```python
from build123d import *

# Parameters (mm, degrees)
F0_W         = 13
F0_H         = 24
F1_DEPTH     = 5
F0_W_2       = 18
F0_H_2       = 5
F2_W         = 83
F2_H         = 80
F3_DEPTH     = 2
F4_W         = 9
F4_H         = 17
F5_DEPTH     = 5
F6_W         = 12
F6_H         = 6
F7_DEPTH     = 10
F8_W         = 12
F8_H         = 4
F9_DEPTH     = 10
F10_T1_DEPTH = 9


# Not quite as in the source:
# - a fillet or chamfer that OpenCascade refuses, or shapes differently, is made with other operations: its cross-section is extruded or revolved along the edge and cut away or added


with BuildPart() as f1:
    # F0 (on Top) → F1 (new body)
    with BuildSketch(Plane.XY):
        Polygon((-19.7103468106, 42.4778270721), (-46.7103468106, 42.4778270721), (-46.7103468106, -37.5221729279), (36.2896531894, -37.5221729279), (36.2896531894, 42.4778270721), (22.2896531894, 42.4778270721), (22.2896531894, 37.4778270721), (31.2896531894, 37.4778270721), (31.2896531894, -32.5221729279), (-23.7103468106, -32.5221729279), (-23.7103468106, 37.4778270721), (-19.7103468106, 37.4778270721), align=None)
        with Locations((-35.2103468106, -3.5221729279)):
            Rectangle(F0_W, F0_H, mode=Mode.SUBTRACT)
    extrude(amount=F1_DEPTH)



with BuildPart() as f1b:
    # F0 (on Top) → F1, piece 2 (new body)
    with BuildSketch(Plane.XY):
        with Locations((-0.7103468106, 39.9778270721)):
            Rectangle(F0_W_2, F0_H_2)
    extrude(amount=F1_DEPTH)


with BuildPart() as f1_1:
    add(f1.part)

    add(f1b.part)  # F3 merges F1b
    # F2 (on face) → F3 (join)
    with BuildSketch(Plane(origin=(0, 0, 0), x_dir=(1, 0, 0), z_dir=(0, 0, -1))):
        with Locations((-5.2103468106, -2.4778270721)):
            Rectangle(F2_W, F2_H)
    extrude(amount=F3_DEPTH)

    # F4 (on face) → F5 (cut)
    with BuildSketch(Plane.XY.offset(5)):
        with Locations((-35.2103468106, -24.0221729279)):
            Rectangle(F4_W, F4_H)
    extrude(amount=-F5_DEPTH, mode=Mode.SUBTRACT)

    # F6 (on face) → F7 (join)
    with BuildSketch(Plane.XY.offset(5)):
        with Locations((-35.2103468106, 11.4778270721)):
            Rectangle(F6_W, F6_H)
    extrude(amount=F7_DEPTH)

    # F8 (on face) → F9 (join)
    with BuildSketch(Plane.XY.offset(5)):
        with Locations((-35.2103468106, -18.5221729279)):
            Rectangle(F8_W, F8_H)
    extrude(amount=F9_DEPTH)

    # F10: fillet of radius 12 on 1 edges, made by hand

    # F10_s2 → F10_t1 (join)
    with BuildSketch(Plane.YZ.offset(-39.7103468106)):
        with BuildLine():
            ThreePointArc((-32.5221729279, 5), (-28.2526041581, 1.322921748), (-22.775378583, 0))
            Line((-22.775378583, 0), (-32.5221729279, 0))
            Line((-32.5221729279, 0), (-32.5221729279, 5))
        make_face()
    extrude(amount=F10_T1_DEPTH)


solid = f1_1.part
```
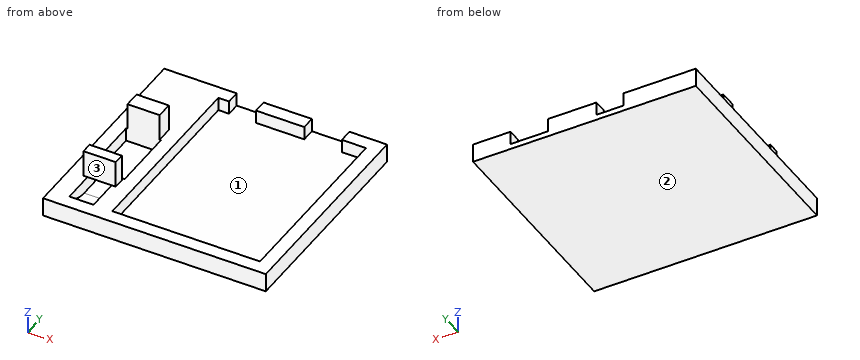
Here's how the part is built. I have some questions about the finished solid (model axes, mm). Face numbers are marked on the shaded views. Coordinates: 2 decimals unless noted, no trailing zeros. Order: outer loops, then holes, each group sorted by start corner. A loop starts at its lowest first (then second) coordinate and runs counter-clockwise, first axis right, second up. Notation, with made-up numbers: (84, 68) - (117, 68) arc R10 ccw to (117, 76) - close; hole circle Ø10 at (46, -32). An arc over 180 degrees is marked (long way). One line per question, with ' | ' between items.
(1) If we mould it in two halves opening along Y, with no side actions, what happens to the marked faces 1, 2 and 3? For each: pulls with the +Y half, pulls with the -Y half, needs draft (parallel to the pull), parting line crosses it, or undercut.
Report:
face 1: undercut | face 2: needs draft | face 3: pulls with the -Y half
(2) Suppose I cut it at C-C on y = 16. List the corners of the cut face in (x, z) for me.
Report:
outline: (-46.71, -2) - (36.29, -2) - (36.29, 5) - (31.29, 5) - (31.29, 0) - (-23.71, 0) - (-23.71, 5) - (-46.71, 5) - close
(3) Suppose I cut it at A-A on y = -17.5. List the corners of the cut face in (x, z) for me.
Report:
outline: (-46.71, -2) - (36.29, -2) - (36.29, 5) - (31.29, 5) - (31.29, 0) - (-23.71, 0) - (-23.71, 5) - (-29.21, 5) - (-29.21, 15) - (-41.21, 15) - (-41.21, 5) - (-46.71, 5) - close; hole (-39.71, 0) - (-30.71, 0) - (-30.71, 5) - (-39.71, 5) - close
(4) Suppose I cut it at D-D on x = 0. List the corners of the cut face in (y, z) for me.
Report:
outline: (-37.52, -2) - (42.48, -2) - (42.48, 5) - (37.48, 5) - (37.48, 0) - (-32.52, 0) - (-32.52, 5) - (-37.52, 5) - close
(5) Suppose I cut it at B-B on z = 6. List the corners of the cut face in (x, y) for me.
Report:
outline: (-41.21, -20.52) - (-29.21, -20.52) - (-29.21, -16.52) - (-41.21, -16.52) - close; (-41.21, 8.48) - (-29.21, 8.48) - (-29.21, 14.48) - (-41.21, 14.48) - close
(6) Will these pins go through, and if not, where does the flat tip stop? pin 1 (1.2 mm diameter, centred on y = -18, z = 8.5, fed in from +X); pin 2 (8 mm diameter, centred on x = -33.5, z = 10.5, fed in from +Y); pin 3 (2 mm diameter, centred on x = -11.5, y = 12, fed in from +Z).
Report:
pin 1: stops at x = -29.21 | pin 2: stops at y = 14.48 | pin 3: stops at z = 0
(7) If I drill on L1, parallel to X at y = -6, z = 1.25; L2, parallel to X at y = -19, z = 4; L3, parallel to X at y = 9, z = 1.75, over which ranges is the centre line in solid material (lowest first)?
Report:
L1: x = -46.71 to -41.71, -28.71 to -23.71, 31.29 to 36.29 | L2: x = -46.71 to -39.71, -30.71 to -23.71, 31.29 to 36.29 | L3: x = -46.71 to -23.71, 31.29 to 36.29
